For this review, take the finished solid that the model builds, in its own axes (mm). A direction names the side the tool comes from. Coordinates: 2 decimals unless noted, no trailing zeros. Loops run counter-clockwise (first coordinate to the right, second up) from the corner with the lowest first, then second, coordinate; pieces in that order, holes last.
```python
from build123d import *

# Parameters (mm, degrees)
F1_DEPTH    = 20
F2_W        = 13
F2_H        = 13
F3_DEPTH    = 40
F4_R        = 2.5
F5_REACH    = 22.0720678119
F6_F1_R     = 3
F6_F2_R     = 3
F7_DEPTH    = 3
F8_T1_DEPTH = 29


# Not quite as in the source:
# - a fillet or chamfer that OpenCascade refuses, or shapes differently, is made with other operations: its cross-section is extruded or revolved along the edge and cut away or added


with BuildPart() as f1:
    # F0 (on Right) → F1 (new body)
    with BuildSketch(Plane.YZ):
        with BuildLine():
            Line((0, -18.2842712475), (0, 0))
            Line((0, 0), (-4.5, 0))
            ThreePointArc((-4.5, 0), (-7.5, -3), (-10.5, 0))
            Line((-10.5, 0), (-15, 0))
            Line((-15, 0), (-15, -5))
            Line((-15, -5), (-43.8908729653, -33.8908729653))
            Line((-43.8908729653, -33.8908729653), (-29.7487373415, -48.033008589))
            Line((-29.7487373415, -48.033008589), (0, -18.2842712475))
        make_face()
    extrude(amount=F1_DEPTH)

    # F2 (on face) → F3 (cut)
    with BuildSketch(Plane(origin=(0, -38.8908729653, -38.8908729653), x_dir=(1, 0, 0), z_dir=(0, -0.7071067812, -0.7071067812))):
        with Locations((10, -2.9289321881)):
            Rectangle(F2_W, F2_H)
    extrude(amount=-F3_DEPTH, mode=Mode.SUBTRACT)

    f5_end = f1.faces().sort_by_distance((10, 0, -9.1421356237))[0]
    # F4 (on face) → F5 (cut, up to a face of the model that its end follows)
    with BuildSketch(Plane(origin=(0, -10.6066017178, -10.6066017178), x_dir=(1, 0, 0), z_dir=(0, -0.7071067812, -0.7071067812))):
        with Locations((10, -2.9289321881)):
            Circle(F4_R)
    f5_long = extrude(amount=-F5_REACH, mode=Mode.PRIVATE)
    add(split(f5_long, bisect_by=f5_end, keep=Keep.BOTTOM, mode=Mode.PRIVATE), mode=Mode.SUBTRACT)

    # F6: fillet of radius 3 on 12 edges, made by hand

    # F6_f1
    f6_f1_edges = [f1.edges().sort_by_distance(p)[0] for p in [
        (10, -15, -5),
    ]]
    fillet(f6_f1_edges, radius=F6_F1_R)

    # F6_f2
    f6_f2_edges = [f1.edges().sort_by_distance(p)[0] for p in [
        (10, -43.8908729653, -33.8908729653),
        (0, -36.8198051534, -40.9619407771),
        (10, -29.7487373415, -48.033008589),
        (20, -36.8198051534, -40.9619407771),
        (10, 0, -18.2842712475),
        (20, -14.8743686708, -33.1586399182),
        (20, 0, -9.1421356237),
        (20, -15, -1.8786796564),
        (0, -15, -1.8786796564),
        (0, -14.8743686708, -33.1586399182),
        (0, 0, -9.1421356237),
        (0, -15.2283614025, -4.90540961),
        (20, -15.2283614025, -4.90540961),
    ]]
    fillet(f6_f2_edges, radius=F6_F2_R)

    # F7 (add): faces of the model
    f7_faces = [f1.faces().sort_by_distance(p)[0] for p in [
        (10, -2.3208506609, 0),
        (10, -12.6791493391, 0),
    ]]
    extrude(f7_faces, amount=F7_DEPTH)

    # F8: fillet of radius 3 on 2 edges, made by hand

    # F8_s2 → F8_t1 (cut)
    with BuildSketch(Plane.YZ.offset(-4.5)):
        with BuildLine():
            ThreePointArc((-15, 0), (-14.1213203436, 2.1213203436), (-12, 3))
            Line((-12, 3), (-15, 3))
            Line((-15, 3), (-15, 0))
        make_face()
        with BuildLine():
            ThreePointArc((-3, 3), (-0.8786796564, 2.1213203436), (0, 0))
            Line((0, 0), (0, 3))
            Line((0, 3), (-3, 3))
        make_face()
    extrude(amount=F8_T1_DEPTH, mode=Mode.SUBTRACT)


solid = f1.part
```
Q1. Wall thickness on probe 1 along X at (y, z) = (-34.5, -32); probe 2 along Y at (x, z) = (7, -22.5); probe 3 along Z at (x, y) = (4, -31.5): over which ranges is each line inside the solid? List them lowest first.
Q2. Machinability: for faces 1 (the face through (10, -15, -2)), 2 (the face through (3.5, -23, -27)), 3 (the face through (0.86, -28.37, -19.64)), which of the approach directions +Z, -Z, +X, -X, +Y, -Y give a long, thin tool a straight path to every point of the face, cutting with its end or side? Answer none if there is none.
Q3. Consider section B-B (x = 8.5). State the section outline as (y, z) points, then the cut area to 3 significant figures.
Q4. For pin 1 Ø6 at (x, y) = (12.5, -34) entering from -Z; pin 2 Ø3.5 at (x, z) = (12, 1.5) entering from -Y; pin 3 Ø1.5 at (x, z) = (10.5, 2) entering from +Y, all flat-tipped, find the tip position at first contact; note any pin that passes through.
Q5. Consider section C-C (x = 18.5). State the section outline as (y, z) points, then the cut area to 3 significant figures.
Q6. Consider section A-A (x = 13.25). State the section outline as (y, z) points, then the cut area to 3 significant figures.
Q7. The part is to be moulded in two halves that separate along Y. For faces 4 (the face through (9.9, -7.4, -3)), 5 (the face through (10.098, -0.235, -18.205)), 6 (the face through (9.91, -27.47, -22.42)), 7 (the face through (0, -19, -22)), say which applies: +Y half, -Y half, draft (parallel to the pull), parting line (faces both ways), or undercut.
Model answer:
1. probe 1: x = 0 to 3.5, 16.5 to 20
1. probe 2: y = -32.5 to -27.55, -9.17 to -4.22
1. probe 3: z = -46.23 to -44.83, -26.45 to -21.5
2. face 1: +Z, +X, -X, -Y
2. face 2: none
2. face 3: +Z, -X, -Y
3. outline: (-41.77, -36.01) - (-41.42, -36.37) - (-13.13, -8.08) - (-9.95, -11.26) - (0, -1.31) - (0, 0) arc R3 ccw to (-3, 3) - (-4.5, 3) - (-4.5, 0) arc R3 cw to (-10.5, 0) - (-10.5, 3) - (-12, 3) arc R3 ccw to (-15, 0) - (-15, -3.76) arc R3 cw to (-15.88, -5.88) - (-41.77, -31.77) arc R3 ccw to start; (-32.22, -45.56) - (-31.87, -45.91) arc R3 ccw to (-27.63, -45.91) - (-0.88, -19.16) arc R3 ccw to (0, -17.04) - (0, -6.97) - (-7.12, -14.09) - (-3.94, -17.27) - close
3. area: 441 mm2
4. pin 1: stops at z = -46.52
4. pin 2: stops at y = -15
4. pin 3: stops at y = -0.27
5. outline: (-41.49, -35.73) - (-31.59, -45.63) arc R2.6 ccw to (-27.91, -45.63) - (-1.16, -18.88) arc R2.6 ccw to (-0.4, -17.04) - (-0.4, 1.5) arc R3 ccw to (-3, 3) - (-4.5, 3) - (-4.5, 0) arc R3 cw to (-10.5, 0) - (-10.5, 3) - (-12, 3) arc R3 ccw to (-14.6, 1.5) - (-14.6, -3.76) arc R3.4 cw to (-15.59, -6.16) - (-41.49, -32.05) arc R2.6 ccw to start
5. area: 959 mm2
6. outline: (-41.77, -36.01) - (-41.42, -36.37) - (-13.13, -8.08) - (-3.94, -17.27) - (-32.22, -45.56) - (-31.87, -45.91) arc R3 ccw to (-27.63, -45.91) - (-0.88, -19.16) arc R3 ccw to (0, -17.04) - (0, 0) arc R3 ccw to (-3, 3) - (-4.5, 3) - (-4.5, 0) arc R3 cw to (-10.5, 0) - (-10.5, 3) - (-12, 3) arc R3 ccw to (-15, 0) - (-15, -3.76) arc R3 cw to (-15.88, -5.88) - (-41.77, -31.77) arc R3 ccw to start
6. area: 489 mm2
7. face 4: undercut
7. face 5: +Y half
7. face 6: undercut
7. face 7: draft
